Input: part model. Units: mm. Frame: model coordinates. A direction names the side the tool comes from. Round coordinates to 2 decimals unless told otherwise and drop trailing zeros. Order: outer loops, then holes, each group sorted by start corner. A loop starts at its lowest first (then second) coordinate and runs counter-clockwise, first axis right, second up. Notation, with made-up numbers: (-2.5, 31) -> (34.5, 31) arc R26 cw to (34.5, 60) -> close; hole circle Ø9 at (65.25, 81.5). An arc over 180 degrees is marked (long way). Use a Markdown table: item, result.
from build123d import *

# Parameters (mm, degrees)
F1_DEPTH    = 30
F3_DEPTH    = 25
F5_T1_DEPTH = 147.1699056603
F6_R        = 1


# Not quite as in the source:
# - a fillet or chamfer that OpenCascade refuses, or shapes differently, is made with other operations: its cross-section is extruded or revolved along the edge and cut away or added


with BuildPart() as f1:
    # F0 (on Right) → F1 (new body)
    with BuildSketch(Plane.YZ):
        Polygon((-25, 0), (0, 0), (0, 40), align=None)
    extrude(amount=F1_DEPTH)

    # F2 (on face) → F3 (cut)
    with BuildSketch(Plane.YZ.offset(30)):
        Polygon((-14.8754669353, 3.6356896162), (0, 3.6356896162), (0, 27.4364367127), align=None)
    extrude(amount=-F3_DEPTH, mode=Mode.SUBTRACT)

    # F4: F1 across face


with BuildPart() as f1_1:
    add(f1.part)
    add(f1.part.mirror(Plane(origin=(30, -10.1830881956, 14.3002167565), x_dir=(0, 1, 0), z_dir=(1, 0, 0))))

    # F5: fillet of radius 5 on 1 edges, made by hand

    # F5_s2 → F5_t1 (cut)
    with BuildSketch(Plane.YZ.offset(-43.5849528301)):
        with BuildLine():
            ThreePointArc((0, 22.5660188679), (-3.6215874348, 27.3722625988), (-9.23999152, 25.216013568))
            Line((-9.23999152, 25.216013568), (0, 40))
            Line((0, 40), (0, 22.5660188679))
        make_face()
    extrude(amount=F5_T1_DEPTH, mode=Mode.SUBTRACT)

    # F6
    f6_edges = [f1_1.edges().sort_by_distance(p)[0] for p in [
        (30, -25, 0),
    ]]
    fillet(f6_edges, radius=F6_R)


solid = f1_1.part
1) Cut plane A-A on x = 21.5. Return loops of the section in (y, z), and give its area (3 significant figures).
Results found:
| item | result |
|---|---|
| outline | (-24.04, 1.53) arc R1 ccw to (-23.2, 0) -> (0, 0) -> (0, 3.64) -> (-14.88, 3.64) -> (-1.09, 25.69) arc R5 ccw to (-9.24, 25.22) -> close |
| area | 269 mm² |
2) Cut plane B-B on y = -7.25. Return loops of the section in (x, z), and give its area (3 significant figures).
Results found:
| item | result |
|---|---|
| outline | (0, 0) -> (60, 0) -> (60, 27.03) -> (0, 27.03) -> close; hole (5, 3.64) -> (55, 3.64) -> (55, 15.84) -> (5, 15.84) -> close |
| area | 1,010 mm² |
3) Pin query (flat end, axial travel): pin 1 Ø6 at (x, z) = (9.5, 16) entering from +Y; pin 2 Ø6 at (x, y) = (38, -20) entering from +Z; pin 3 Ø1 at (x, y) = (32.5, -12.5) entering from +Z; pin 4 Ø12 at (x, y) = (18, -7) entering from +Z. Return the tip coordinate at first contact, or that it passes through.
Results found:
| item | result |
|---|---|
| pin 1 | stops at y = -5.27 |
| pin 2 | stops at z = 12.8 |
| pin 3 | stops at z = 20.8 |
| pin 4 | stops at z = 27.57 |
4) Pull-direction query (Z, two-part tool) for faces 3 (the flat face through (30, -12, 0)), 4 (the flat face through (30.42, -16.538, 13.539)), 5 (the flat face through (5, -4, 12)), 6 (the flat face through (30, 0, 1)); classes: +Z half, -Z half, draft (parallel to the pull), parting line (faces both ways), or undercut.
Results found:
| item | result |
|---|---|
| face 3 | -Z half |
| face 4 | +Z half |
| face 5 | undercut |
| face 6 | draft |
5) Cut plane D-D on y = -21. Return loops of the section in (x, z).
Results found:
| item | result |
|---|---|
| outline | (0, 0) -> (60, 0) -> (60, 6.4) -> (0, 6.4) -> close |
6) Line query: L1, parallel to X at y = -4.5, z = 5; L2, parallel to Z at x = 19, y = -2.25; L3, parallel to Z at x = 13.5, y = -6.25. Output: solid intervals per line, ascending. Write a range as [from, to].
Results found:
| item | result |
|---|---|
| L1 | x = [0, 5], [55, 60] |
| L2 | z = [0, 3.64], [23.84, 26.74] |
| L3 | z = [0, 3.64], [17.44, 27.41] |
7) Cut plane C-C on z = 13.5. Return loops of the section in (x, y).
Results found:
| item | result |
|---|---|
| outline | (0, -16.56) -> (60, -16.56) -> (60, 0) -> (55, 0) -> (55, -8.71) -> (5, -8.71) -> (5, 0) -> (0, 0) -> close |
8) Set-up query: faces 1 (the flat face through (0, -10, 11)), 2 (the flat face through (29.6, -7.9, 14.8)). Return all of +Z, -Z, +X, -X, +Y, -Y with unobstructed straight access to the full face (end or side cutting, diameter ignored); none if empty.
Results found:
| item | result |
|---|---|
| face 1 | +Z, -Z, -X, +Y, -Y |
| face 2 | +Y |
